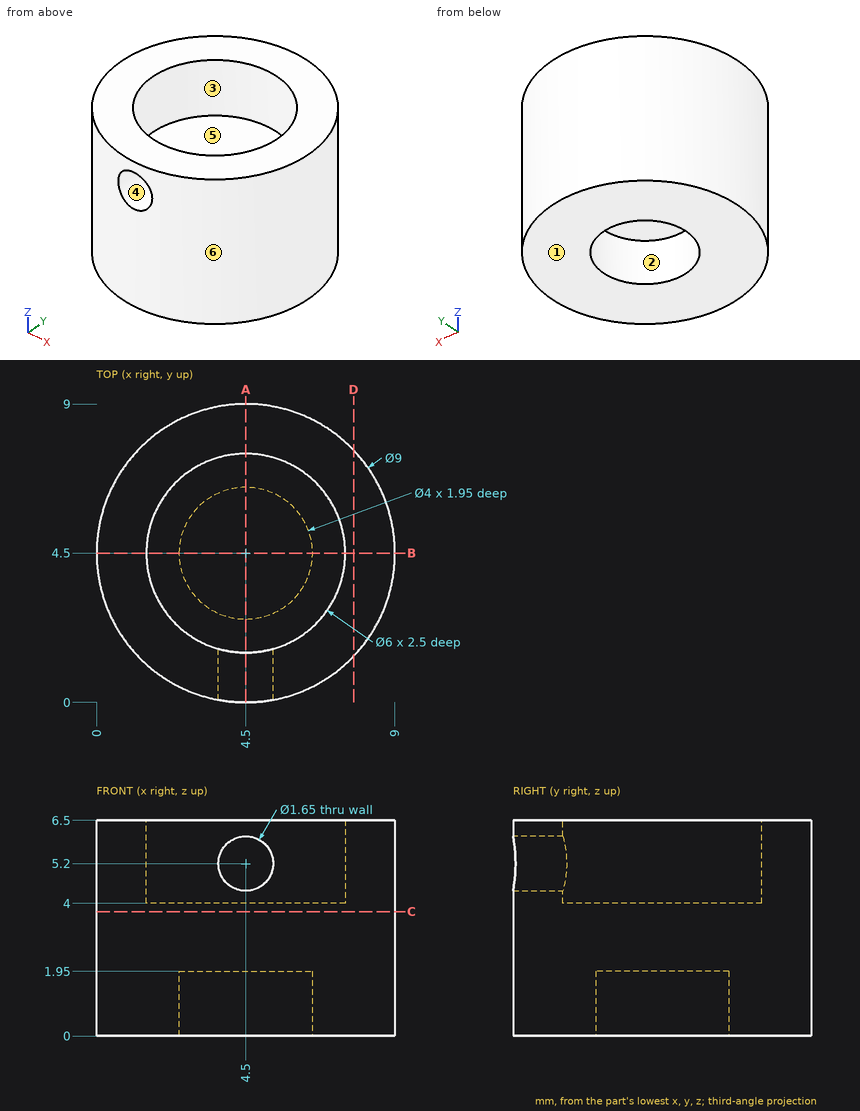
Geometry: see drawing. Coordinates: mm, zero at the bounding-box minimum. A direction names the side the tool comes from. Round coordinates to 2 decimals unless told otherwise and drop trailing zeros. Order: outer loops, then holes, each group sorted by start corner. A loop starts at its lowest first (then second) coordinate and runs counter-clockwise, first axis right, second up. Notation, with made-up numbers: (-34.5, 26.5) -> (18.5, 26.5) arc R20 ccw to (18.5, 40.5) -> close; hole circle Ø3 at (-32.5, 30). An arc over 180 degrees is marked (long way). Use CSV: the item, a comma, the result in double quotes.
(1) Access query for the marked faces 1, 2 and 3. Directions: +Z, -Z, +X, -X, +Y, -Y. A direction counts if a zero-diameter tool reaches every point of the face in a straight line with its end or side. Return the directions, or none.
Report:
face 1,"-Z, +X, -X, +Y, -Y"
face 2,"-Z"
face 3,"+Z"
(2) Ray query, L1, parallel to Y at x = 4.5, z = 1.25; L2, parallel to Y at x = 4.5, z = 4.75; L3, parallel to Z at x = 4.75, y = 2.75. Return the intervals inside material, ascending.
Report:
L1,"0 to 2.5, 6.5 to 9"
L2,"7.5 to 9"
L3,"1.95 to 4"
(3) Pull-direction query (Y, two-part tool) for the marked faces 4, 5 and 6; classes: +Y half, -Y half, draft (parallel to the pull), parting line (faces both ways), or undercut.
Report:
face 4,"draft"
face 5,"undercut"
face 6,"parting line"
(4) First-contact query: pin 1 Ø1 at (x, y) = (4.5, 4.5) entering from +Z; pin 2 Ø1.5 at (x, z) = (5.5, 4) entering from +Y; pin 3 Ø1.5 at (x, z) = (4.5, 5.2) entering from -Y. Flat tips, straight axial feed; report the tip coordinate or a pass-through.
Report:
pin 1,"z = 4"
pin 2,"y = 8.99"
pin 3,"y = 7.4"
(5) Section B-B on y = 4.5. Return the cut outline in (x, z).
Report:
outline,"(0, 0) -> (2.5, 0) -> (2.5, 1.95) -> (6.5, 1.95) -> (6.5, 0) -> (9, 0) -> (9, 6.5) -> (7.5, 6.5) -> (7.5, 4) -> (1.5, 4) -> (1.5, 6.5) -> (0, 6.5) -> close"
(6) Section C-C on z = 3.75. Return the cut outline in (x, y), and give its area (3 significant figures).
Report:
outline,"circle Ø9 at (4.5, 4.5)"
area,"63.6 mm^2"
(7) Section A-A on x = 4.5. Return the cut outline in (y, z) (3 decimals), and give its area (3 significant figures).
Report:
outline,"(0, 0) -> (2.5, 0) -> (2.5, 1.95) -> (6.5, 1.95) -> (6.5, 0) -> (9, 0) -> (9, 6.5) -> (7.5, 6.5) -> (7.5, 4) -> (1.5, 4) -> (1.5, 4.375) -> (0, 4.375) -> close; (0, 6.025) -> (1.5, 6.025) -> (1.5, 6.5) -> (0, 6.5) -> close"
area,"33.2 mm^2"
(8) Section D-D on x = 7.75. Return the cut outline in (y, z).
Report:
outline,"(1.39, 0) -> (7.61, 0) -> (7.61, 6.5) -> (1.39, 6.5) -> close"
